Build history of the part. All positions in model axes, mm. A direction names the side the tool comes from. Give positions to 0.01 mm unless a question says otherwise; leave off trailing zeros. Write each loop counter-clockwise with the first axis right and the second up, starting at its lowest first coordinate (ties: lowest second). Pieces come first, ordered by that corner, then holes. Notation, with made-up numbers: M -38,33 L -19,33 A18 cw -19,53 Z; hole C 61.5,44.5 d7. An arc over 180 degrees is marked long. One line per item, written item: value. Start each with the question number.
Autodesk Inventor part; units mm, degrees
ref_plane "YZ Plane" through (0, 0, 0) normal (1, 0, 0) x (0, 1, 0)
ref_plane "XZ Plane" through (0, 0, 0) normal (0, 1, 0) x (-1, 0, 0)
ref_plane "XY Plane" through (0, 0, 0) normal (0, 0, 1) x (1, 0, 0)
sketch "Sketch1" plane through (0, 0, 0) normal (0, 0, 1) x (1, 0, 0)
  circle A0 centre (0, 0) radius 1.5
  dimension "d0" = 3
extrude "Extrusion1" add sketch "Sketch1" along normal blind 3
chamfer "Chamfer1" distance 0.25 angle 45 2 edges at (-1.5, 0, 3) (-1.5, 0, 0)
sketch "Sketch2" plane through (0, 0, 3) normal (0, 0, 1) x (1, 0, 0)
  circle A0 centre (0, 0) radius 0.6
  dimension "d12" = 1.2
extrude "Extrusion2" add sketch "Sketch2" along normal blind 1.5
fillet "Fillet1" radius 0.5 1 edges at (-0.6, 0, 4.5)
sketch "Sketch3" plane through (0, 0, 0) normal (0, 0, -1) x (-1, 0, 0)
  circle A0 centre (0, 0) radius 0.15
  dimension "d9" = 0.3
extrude "Extrusion3" add sketch "Sketch3" along normal blind 3
properties part number "DC motor"
1) Probe line 1 along Z through (x, y) = (-0.5, -0.9); line 2 along X through (y, z) = (0.5, 2.5); line 3 along Z through (x, y) = (0.9, -1.1). List the from-to ranges inside material, lowest first. Write a range as from..to.
2) Band-saw the part on B-B (z = 1.5). List the corners of the cut face in (x, y), then the cut area to 3 significant figures.
3) Band-saw the part on A-A (z = -2.25). List the corners of the cut face in (x, y).
4) Drop a flat-ended pin along its axis: P1, Ø1, axis at x = 1, z = 0, coming from the +Y side. Give the stop position or say it passes through.
5) Tool access for faces 1 (the face through (-1.5, -0.07, 1.48)), 2 (the face through (0.323, -0.506, 3.493)): list every direction of +Z, -Z, +X, -X, +Y, -Y with a clear straight run to the whole face (end or side of a thin tool).
Model answer:
1. line 1: z = 0..3
1. line 2: x = -1.41..1.41
1. line 3: z = 0.17..2.83
2. outline: C 0,0 d3
2. area: 7.07 mm²
3. outline: C 0,0 d0.3
4. P1: stops at y = 1.39
5. face 1: +Z, -Z
5. face 2: +Z
